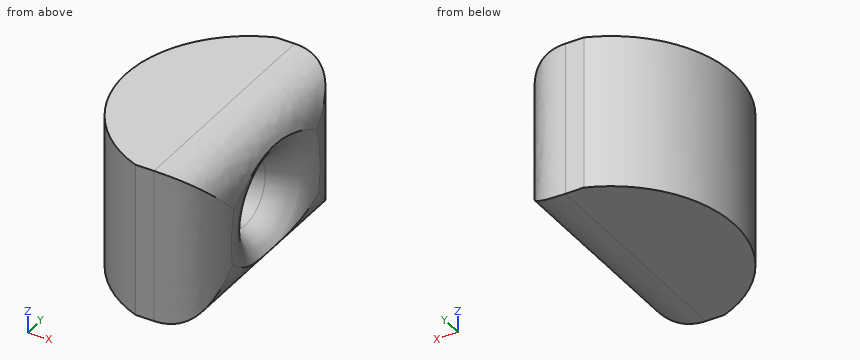
from build123d import *

# Parameters (mm, degrees)
F1_DEPTH    = 47.244
F2_R        = 13.7417577373
F4_T1_DEPTH = 123.444
F4_T3_DEPTH = 147.3045786738


# Not quite as in the source:
# - a fillet or chamfer that OpenCascade refuses, or shapes differently, is made with other operations: its cross-section is extruded or revolved along the edge and cut away or added
# - an extrude whose draft closes it to a point is written as a loft to that point


with BuildPart() as f1:
    # F0 (on Top) → F1 (new body)
    with BuildSketch(Plane.XY):
        with BuildLine():
            Line((-38.2979549468, 31.997974962), (-59.2006028914, 31.997974962))
            ThreePointArc((-59.2006028914, 31.997974962), (-83.8900545196, -3.5543143749), (-59.2006028914, -39.1066037118))
            Line((-59.2006028914, -39.1066037118), (-38.2979549468, -39.1066037118))
            Line((-38.2979549468, -39.1066037118), (-38.2979549468, 31.997974962))
        make_face()
    extrude(amount=F1_DEPTH)

    # F2 (on face) → F3 section 0
    with BuildSketch(Plane.YZ.offset(-38.2979549468), mode=Mode.PRIVATE) as f3_s0:
        with Locations((-1.4992692741, 20.8444874734)):
            Circle(F2_R)
    loft([f3_s0.sketch, Vertex(-76.0531240335, -1.4992692741, 20.8444874734)], ruled=True, mode=Mode.SUBTRACT)

    # F4: fillet of radius 15.24 on 5 edges, made by hand

    # F4_s2 → F4_t1 (cut)
    with BuildSketch(Plane.XY.offset(-38.1)):
        with BuildLine():
            add(Edge.make_bspline(
                [(-53.5379549468, -39.1066037118), (-38.2979549468, -39.1066037118), (-38.2979549468, -23.8666037118)],
                knots=[0, 0, 0, 1, 1, 1], degree=2, weights=[1, 1, 1]))
            Line((-38.2979549468, -23.8666037118), (-38.2979549468, -39.1066037118))
            Line((-38.2979549468, -39.1066037118), (-53.5379549468, -39.1066037118))
        make_face()
        with BuildLine():
            add(Edge.make_bspline(
                [(-53.5379549468, 31.997974962), (-38.2979549468, 31.997974962), (-38.2979549468, 16.757974962)],
                knots=[0, 0, 0, 1, 1, 1], degree=2, weights=[1, 1, 1]))
            Line((-38.2979549468, 16.757974962), (-38.2979549468, 31.997974962))
            Line((-38.2979549468, 31.997974962), (-53.5379549468, 31.997974962))
        make_face()
    extrude(amount=F4_T1_DEPTH, mode=Mode.SUBTRACT)

    # F4_s4 → F4_t3 (cut)
    with BuildSketch(Plane.XZ.offset(-70.097974962)):
        with BuildLine():
            add(Edge.make_bspline(
                [(-53.5379549468, 0), (-38.2979549468, 0), (-38.2979549468, 15.24)],
                knots=[0, 0, 0, 1, 1, 1], degree=2, weights=[1, 1, 1]))
            Line((-38.2979549468, 15.24), (-38.2979549468, 0))
            Line((-38.2979549468, 0), (-53.5379549468, 0))
        make_face()
        with BuildLine():
            add(Edge.make_bspline(
                [(-53.5379549468, 47.244), (-38.2979549468, 47.244), (-38.2979549468, 32.004)],
                knots=[0, 0, 0, 1, 1, 1], degree=2, weights=[1, 1, 1]))
            Line((-38.2979549468, 32.004), (-38.2979549468, 47.244))
            Line((-38.2979549468, 47.244), (-53.5379549468, 47.244))
        make_face()
    extrude(amount=F4_T3_DEPTH, mode=Mode.SUBTRACT)

    # F4_s5 → F4_t6 (revolve, cut)
    with BuildSketch(Plane.XY.offset(20.8444874734)):
        with BuildLine():
            add(Edge.make_bspline(
                [(-38.2979549468, 22.9136513455), (-38.2979549468, 12.2424884632), (-48.3255679625, 8.5927358047)],
                knots=[0, 0, 0, 1, 1, 1], degree=2, weights=[1, 1, 1]))
            Line((-48.3255679625, 8.5927358047), (-38.2979549468, 12.2424884632))
            Line((-38.2979549468, 12.2424884632), (-38.2979549468, 22.9136513455))
        make_face()
    revolve(axis=Axis((-38.2979549468, -1.4992692741, 20.8444874734), (1, 0, 0)), mode=Mode.SUBTRACT)


solid = f1.part
Source: CAD feature listing. Evaluate the final solid. Frame: model axes, mm. Coordinates: 2 decimals unless noted, no trailing zeros. Loops run counter-clockwise (first coordinate to the right, second up) from the corner with the lowest first, then second, coordinate; pieces in that order, holes last. Notation, with made-up numbers: (59, 64.5) - (96, 64.5) arc R20 ccw to (96, 70.5) - close; hole circle Ø11 at (11.25, -9). An arc over 180 degrees is marked (long way). One line per item, written item: value. Start each with the question number.
1. Contact query for flat-ended pins moving along their axis: P1, Ø1.5, axis at x = -71, z = 6.5, coming from the +Y side; P2, Ø6, axis at y = 11, z = 15, coming from the +X side; P3, Ø8, axis at x = -76, z = 36, coming from the -Y side. Output: stop coordinate, or through.
2. Ray query, L1, parallel to Z at x = -53, y = -2; L2, parallel to Z at x = -60, y = -6.5; L3, parallel to Y at x = -64.5, z = 24. Return the intervals inside material, ascending.
3. Section A-A (x = -60). Return the cut outline in (y, z), and give its area (3 significant figures).
4. Section B-B (x = -72). Return the cut outline in (y, z), and give its area (3 significant figures).
Verdict:
1. P1: stops at y = 25.58
1. P2: stops at x = -40.01
1. P3: stops at y = -31.14
2. L1: z = 0 to 12.47, 29.22 to 47.24
2. L2: z = 0 to 17.82, 23.87 to 47.24
2. L3: y = -36.65 to -4.28, 1.28 to 29.54
3. outline: (-38.8, 0) - (31.69, 0) - (31.69, 47.24) - (-38.8, 47.24) - close; hole circle Ø11.69 at (-1.5, 20.84)
3. area: 3,220 mm2
4. outline: (-31.14, 0) - (24.03, 0) - (24.03, 47.24) - (-31.14, 47.24) - close; hole circle Ø2.95 at (-1.5, 20.84)
4. area: 2,600 mm2
